from build123d import *

# Parameters (mm, degrees)
SKETCH2_W           = 590
SKETCH2_H           = 279.33
BOSS_EXTRUDE1_DEPTH = 25
CUT_EXTRUDE1_DEPTH  = 22


with BuildPart() as part:
    # Sketch2 → Boss-Extrude1 (new body)
    with BuildSketch(Plane.XY):
        Rectangle(SKETCH2_W, SKETCH2_H)
    extrude(amount=BOSS_EXTRUDE1_DEPTH)

    # Sketch4 → Cut-Extrude1 (cut)
    with BuildSketch(Plane.XY.offset(25)):
        with BuildLine():
            Line((-261, 47.335), (-277.893878125, 47.335))
            ThreePointArc((-277.893878125, 47.335), (-279.344157467, 46.712203627), (-279.891208095, 45.231689829))
            Line((-279.891208095, 45.231689829), (-272.5, -97.665))
            Line((-272.5, -97.665), (-217.5, -97.665))
            Line((-217.5, -97.665), (-210.108791905, 45.231689829))
            ThreePointArc((-210.108791905, 45.231689829), (-210.655842533, 46.712203627), (-212.106121875, 47.335))
            Line((-212.106121875, 47.335), (-229, 47.335))
            Line((-229, 47.335), (-229, 92.335))
            Line((-229, 92.335), (-261, 92.335))
            Line((-261, 92.335), (-261, 47.335))
        make_face()
        with BuildLine():
            Line((-21.456483238, -97.665), (-14.065275143, 45.231689829))
            ThreePointArc((-14.065275143, 45.231689829), (-14.612325771, 46.712203627), (-16.062605113, 47.335))
            Line((-16.062605113, 47.335), (-32.956483238, 47.335))
            Line((-32.956483238, 47.335), (-32.956483238, 92.335))
            Line((-32.956483238, 92.335), (-64.956483238, 92.335))
            Line((-64.956483238, 92.335), (-64.956483238, 47.335))
            Line((-64.956483238, 47.335), (-81.850361363, 47.335))
            ThreePointArc((-81.850361363, 47.335), (-83.300640705, 46.712203627), (-83.847691332, 45.231689829))
            Line((-83.847691332, 45.231689829), (-76.456483238, -97.665))
            Line((-76.456483238, -97.665), (-21.456483238, -97.665))
        make_face()
        with BuildLine():
            Line((-181.869449714, 45.231689829), (-174.478241619, -97.665))
            Line((-174.478241619, -97.665), (-119.478241619, -97.665))
            Line((-119.478241619, -97.665), (-112.087033524, 45.231689829))
            ThreePointArc((-112.087033524, 45.231689829), (-112.634084152, 46.712203627), (-114.084363494, 47.335))
            Line((-114.084363494, 47.335), (-130.978241619, 47.335))
            Line((-130.978241619, 47.335), (-130.978241619, 92.335))
            Line((-130.978241619, 92.335), (-162.978241619, 92.335))
            Line((-162.978241619, 92.335), (-162.978241619, 47.335))
            Line((-162.978241619, 47.335), (-179.872119744, 47.335))
            ThreePointArc((-179.872119744, 47.335), (-181.322399086, 46.712203627), (-181.869449714, 45.231689829))
        make_face()
        with BuildLine():
            Line((76.565275143, -97.665), (83.956483238, 45.231689829))
            ThreePointArc((83.956483238, 45.231689829), (83.40943261, 46.712203627), (81.959153268, 47.335))
            Line((81.959153268, 47.335), (65.065275143, 47.335))
            Line((65.065275143, 47.335), (65.065275143, 92.335))
            Line((65.065275143, 92.335), (33.065275143, 92.335))
            Line((33.065275143, 92.335), (33.065275143, 47.335))
            Line((33.065275143, 47.335), (16.171397019, 47.335))
            ThreePointArc((16.171397019, 47.335), (14.721117676, 46.712203627), (14.174067049, 45.231689829))
            Line((14.174067049, 45.231689829), (21.565275143, -97.665))
            Line((21.565275143, -97.665), (76.565275143, -97.665))
        make_face()
        with BuildLine():
            Line((174.587033524, -97.665), (181.978241619, 45.231689829))
            ThreePointArc((181.978241619, 45.231689829), (181.431190991, 46.712203627), (179.980911649, 47.335))
            Line((179.980911649, 47.335), (163.087033524, 47.335))
            Line((163.087033524, 47.335), (163.087033524, 92.335))
            Line((163.087033524, 92.335), (131.087033524, 92.335))
            Line((131.087033524, 92.335), (131.087033524, 47.335))
            Line((131.087033524, 47.335), (114.1931554, 47.335))
            ThreePointArc((114.1931554, 47.335), (112.742876057, 46.712203627), (112.19582543, 45.231689829))
            Line((112.19582543, 45.231689829), (119.587033524, -97.665))
            Line((119.587033524, -97.665), (174.587033524, -97.665))
        make_face()
        with BuildLine():
            Line((210.217583811, 45.231689829), (217.608791905, -97.665))
            Line((217.608791905, -97.665), (272.608791905, -97.665))
            Line((272.608791905, -97.665), (280, 45.231689829))
            ThreePointArc((280, 45.231689829), (279.452949372, 46.712203627), (278.00267003, 47.335))
            Line((278.00267003, 47.335), (261.108791905, 47.335))
            Line((261.108791905, 47.335), (261.108791905, 92.335))
            Line((261.108791905, 92.335), (229.108791905, 92.335))
            Line((229.108791905, 92.335), (229.108791905, 47.335))
            Line((229.108791905, 47.335), (212.214913781, 47.335))
            ThreePointArc((212.214913781, 47.335), (210.764634438, 46.712203627), (210.217583811, 45.231689829))
        make_face()
    extrude(amount=-CUT_EXTRUDE1_DEPTH, mode=Mode.SUBTRACT)


solid = part.part
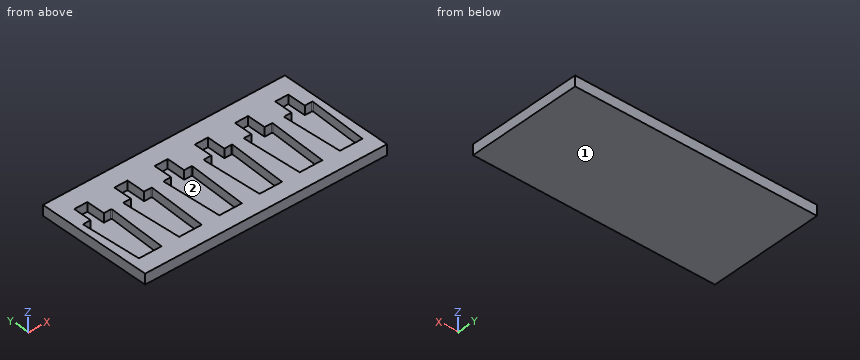
Work out the finished part from the listing and answer in its coordinate system (mm). Face numbers are marked on the shaded views. Give positions to 0.01 mm unless a question says otherwise; leave off trailing zeros. Order: outer loops, then holes, each group sorted by start corner. A loop starts at its lowest first (then second) coordinate and runs counter-clockwise, first axis right, second up. Notation, with made-up numbers: (39, -16) -> (76, -16) arc R34 cw to (76, 14) -> close; hole circle Ø1 at (17, 44.25). An arc over 180 degrees is marked (long way). One line per item, written item: value.
Item 1: Find section B-B, the plane y = 63. Give the vertices of the cut face in (x, z), plus the area to 3 significant figures.
Answer sheet:
outline: (-295, 0) -> (295, 0) -> (295, 25) -> (261.11, 25) -> (261.11, 3) -> (229.11, 3) -> (229.11, 25) -> (163.09, 25) -> (163.09, 3) -> (131.09, 3) -> (131.09, 25) -> (65.07, 25) -> (65.07, 3) -> (33.07, 3) -> (33.07, 25) -> (-32.96, 25) -> (-32.96, 3) -> (-64.96, 3) -> (-64.96, 25) -> (-130.98, 25) -> (-130.98, 3) -> (-162.98, 3) -> (-162.98, 25) -> (-229, 25) -> (-229, 3) -> (-261, 3) -> (-261, 25) -> (-295, 25) -> close
area: 10,500 mm²
Item 2: Determine the mould class of the marked faces 1 and 2 for opening direction X: released by +X, released by -X, zero draft, split by the parting line, or undercut.
Answer sheet:
face 1: zero draft
face 2: undercut
Item 3: Find section D-D, the plane y = 34.5. Give the vertices of the cut face in (x, z).
Answer sheet:
outline: (-295, 0) -> (295, 0) -> (295, 25) -> (279.44, 25) -> (279.44, 3) -> (210.77, 3) -> (210.77, 25) -> (181.42, 25) -> (181.42, 3) -> (112.75, 3) -> (112.75, 25) -> (83.4, 25) -> (83.4, 3) -> (14.73, 3) -> (14.73, 25) -> (-14.62, 25) -> (-14.62, 3) -> (-83.29, 3) -> (-83.29, 25) -> (-112.64, 25) -> (-112.64, 3) -> (-181.31, 3) -> (-181.31, 25) -> (-210.66, 25) -> (-210.66, 3) -> (-279.34, 3) -> (-279.34, 25) -> (-295, 25) -> close
Item 4: A flat-ended cylindrical pin translates along its axis: P1, Ø5, axis at x = -149.5, y = -72.5, coming from the +Z side. Find the tip coordinate at first contact, or state that the pin passes through.
Answer sheet:
P1: z = 3
Item 5: Find section A-A, the plane x = 247.5. Give the vertices of the cut face in (y, z) (3 decimals).
Answer sheet:
outline: (-139.665, 0) -> (139.665, 0) -> (139.665, 25) -> (92.335, 25) -> (92.335, 3) -> (-97.665, 3) -> (-97.665, 25) -> (-139.665, 25) -> close
Item 6: Find section C-C, the plane z = 12. State how many separate pieces and enclosed holes the cut face has, plus the area to 3 significant figures.
Answer sheet:
separate pieces: 1
enclosed holes: 6
area: 102,000 mm²
Item 7: Straight lines are drawn through the part: probe 1 along Y at (x, z) = (-167, 15.25) (3 decimals); probe 2 along Z at (x, y) = (-163, -81.5); probe 3 along Y at (x, z) = (-33, 12) (3 decimals). For each, find the intervals that lie inside material, in ascending order.
Answer sheet:
probe 1: -139.665 to -97.665, 47.335 to 139.665
probe 2: 0 to 3
probe 3: -139.665 to -97.665, 92.335 to 139.665
